from build123d import *

# Parameters (mm, degrees)
F0_W      = 7
F0_H      = 7
F1_DEPTH  = 10
F2_W      = 7
F2_H      = 7
F3_DEPTH  = 30
F4_W      = 52.018345
F4_H      = 10
F5_DEPTH  = 5
F6_W      = 52.018345
F6_H      = 5
F7_DEPTH  = 16
F8_W      = 36
F8_H      = 16
F9_DEPTH  = 25
F10_DEPTH = 25


with BuildPart() as f1:
    # F0 (on Top) → F1 (new body)
    with BuildSketch(Plane.XY):
        Polygon((65.849743, 2.373854), (65.849743, 22.373854), (55.849743, 22.373854), (48.849743, 22.373854), (12.849743, 22.373854), (5.849743, 22.373854), (-4.150257, 22.373854), (-4.150257, 2.373854), align=None)
        with Locations((52.349743, 25.873854)):
            Rectangle(F0_W, F0_H)
        with Locations((9.349743, 25.873854)):
            Rectangle(F0_W, F0_H)
    extrude(amount=F1_DEPTH)

    # F2 (on face) → F3 (join)
    with BuildSketch(Plane.XY.offset(10)):
        with Locations((9.349743, 25.873854)):
            Rectangle(F2_W, F2_H)
        with Locations((52.349743, 25.873854)):
            Rectangle(F2_W, F2_H)
    extrude(amount=F3_DEPTH)

    # F4 (on face) → F5 (join)
    with BuildSketch(Plane.XZ.offset(-2.373854)):
        with Locations((30.946101, 5)):
            Rectangle(F4_W, F4_H)
    extrude(amount=F5_DEPTH)

    # F6 (on face) → F7 (join)
    with BuildSketch(Plane.XY.offset(10)):
        with Locations((30.946101, -0.126146)):
            Rectangle(F6_W, F6_H)
    extrude(amount=F7_DEPTH)

    # F8 (on face) → F9 (cut)
    with BuildSketch(Plane.XZ.offset(2.626146)):
        with Locations((30.849743, 18)):
            Rectangle(F8_W, F8_H)
    extrude(amount=-F9_DEPTH, mode=Mode.SUBTRACT)

    # F8 (on face) → F10 (cut)
    with BuildSketch(Plane.XZ.offset(2.626146)):
        with Locations((30.849743, 18)):
            Rectangle(F8_W, F8_H)
    extrude(amount=-F10_DEPTH, mode=Mode.SUBTRACT)


solid = f1.part
Design review of the part built by this model. Coordinates are the model's own, in mm. A direction names the side the tool comes from. Round coordinates to 2 decimals unless told otherwise and drop trailing zeros. Write each loop counter-clockwise with the first axis right and the second up, starting at its lowest first coordinate (ties: lowest second). Pieces come first, ordered by that corner, then holes. Notation, with made-up numbers: (68, 84) - (101, 84) arc R36 ccw to (101, 118) - close; hole circle Ø8 at (31, 52). An arc over 180 degrees is marked (long way). Return JSON: item names as keys, results as strings. Group by question number.
Item 1: We need section D-D on z = 7. Write out the cut boundary in (x, y).
Item 2: For probe 1 along X at (y, z) = (26, 6.5); probe 2 along Z at (x, y) = (43.5, 7); probe 3 along Y at (x, z) = (1, 3.5), list the stretches that pass through material, from the lowest coordinate up. Write a range as [from, to].
Item 3: We need section A-A on z = 20.5. Write out the cut boundary in (x, y).
Item 4: Machinability: for faces 1 (the face through (56.955, 0, 13)), 2 (the face through (31, 22.374, 5)), 3 (the face through (9, 0, 26)), which of the approach directions +Z, -Z, +X, -X, +Y, -Y give a long, thin tool a straight path to every point of the face, cutting with its end or side? Answer none if there is none.
Item 5: We need section C-C on y = 0.5. Write out the cut boundary in (x, z), and give its area (3 significant figures).
Item 6: Insertion check: P1, Ø1.5, axis at y = 1.5, z = 19, coming from the -X side; P2, Ø6, axis at x = 29.5, z = 7.5, coming from the +Y side; P3, Ø10, axis at x = 63.5, z = 3, coming from the -Y side; P4, Ø2, axis at x = 48.5, z = 17, coming from the +Y side. Each pin has a flat end and moves straight along its axis. Give the tip position at first contact, or say it passes through.
Item 7: We need section B-B on z = 27.5. Write out the cut boundary in (x, y), and give its area (3 significant figures).
Model answer:
{
 "1": {"outline": "(-4.15, 2.37) - (4.94, 2.37) - (4.94, -2.63) - (56.96, -2.63) - (56.96, 2.37) - (65.85, 2.37) - (65.85, 22.37) - (55.85, 22.37) - (55.85, 29.37) - (48.85, 29.37) - (48.85, 22.37) - (12.85, 22.37) - (12.85, 29.37) - (5.85, 29.37) - (5.85, 22.37) - (-4.15, 22.37) - close"},
 "2": {"probe 1": "x = [5.85, 12.85], [48.85, 55.85]", "probe 2": "z = [0, 10]", "probe 3": "y = [2.37, 22.37]"},
 "3": {"outline": "(4.94, -2.63) - (12.85, -2.63) - (12.85, 2.37) - (4.94, 2.37) - close; (5.85, 22.37) - (12.85, 22.37) - (12.85, 29.37) - (5.85, 29.37) - close; (48.85, -2.63) - (56.96, -2.63) - (56.96, 2.37) - (48.85, 2.37) - close; (48.85, 22.37) - (55.85, 22.37) - (55.85, 29.37) - (48.85, 29.37) - close"},
 "4": {"face 1": "+Z, -Z, +X, -Y", "face 2": "+Z, -Z, +Y", "face 3": "+Z, +X, -X, -Y"},
 "5": {"outline": "(4.94, 0) - (56.96, 0) - (56.96, 26) - (48.85, 26) - (48.85, 10) - (12.85, 10) - (12.85, 26) - (4.94, 26) - close", "area": "776 mm²"},
 "6": {"P1": "stops at x = 4.94", "P2": "stops at y = 22.37", "P3": "stops at y = 2.37", "P4": "stops at y = 29.37"},
 "7": {"outline": "(5.85, 22.37) - (12.85, 22.37) - (12.85, 29.37) - (5.85, 29.37) - close; (48.85, 22.37) - (55.85, 22.37) - (55.85, 29.37) - (48.85, 29.37) - close", "area": "98.0 mm²"}
}
